```python
from build123d import *

# Parameters (mm, degrees)
F0_W     = 125
F0_H     = 75
F1_DEPTH = 2
F2_W     = 125
F2_H     = 2
F3_DEPTH = 40
F4_R     = 5
F5_R     = 5.08
F6_DEPTH = 100


with BuildPart() as f1:
    # F0 (on Front) → F1 (new body)
    with BuildSketch(Plane.XZ):
        Rectangle(F0_W, F0_H)
    extrude(amount=F1_DEPTH)

    # F2 (on face) → F3 (join)
    with BuildSketch(Plane.XZ.offset(2)):
        with Locations((0, -36.5)):
            Rectangle(F2_W, F2_H)
        with Locations((0, 36.5)):
            Rectangle(F2_W, F2_H)
    extrude(amount=F3_DEPTH)

    # F4
    f4_edges = [f1.edges().sort_by_distance(p)[0] for p in [
        (0, 0, 37.5),
        (0, 0, -37.5),
    ]]
    fillet(f4_edges, radius=F4_R)

    # F5 (on face) → F6 (cut)
    with BuildSketch(Plane.XY.offset(37.5)):
        with Locations((37.42, -25.08)):
            Circle(F5_R)
        with Locations((-37.42, -25.08)):
            Circle(F5_R)
    extrude(amount=-F6_DEPTH, mode=Mode.SUBTRACT)


solid = f1.part
```
Design review of the part built by this model. Coordinates are the model's own, in mm. A direction names the side the tool comes from. Give positions to 0.01 mm unless a question says otherwise; leave off trailing zeros. Write each loop counter-clockwise with the first axis right and the second up, starting at its lowest first coordinate (ties: lowest second). Pieces come first, ordered by that corner, then holes.
(1) Add section D-D (x = -2.5). Give the boundary of the cut face in (y, z), and give its area (3 significant figures).
Checked values:
outline: (-42, -37.5) - (-5, -37.5) arc R5 ccw to (0, -32.5) - (0, 32.5) arc R5 ccw to (-5, 37.5) - (-42, 37.5) - (-42, 35.5) - (-2, 35.5) - (-2, -35.5) - (-42, -35.5) - close
area: 299 mm2
(2) Tool access review of faces 4 (the face through (-1, -22, -35.5)), 5 (the face through (40.151, -20.797, -36.486)): name each direction out of +Z, -Z, +X, -X, +Y, -Y from which nothing blocks a thin tool from reaching the whole face with its end or side.
Checked values:
face 4: +X, -X, -Y
face 5: +Z, -Z
(3) Clearance check with flat-ended pins moving along their axes: pin 1 Ø13 at (x, y) = (-37.42, -25.08) entering from -Z; pin 2 Ø21.5 at (x, z) = (-22.5, -17) entering from -Y; pin 3 Ø8 at (x, y) = (-37.42, -25.08) entering from -Z. State where each tip first meets the part, or that it passes through.
Checked values:
pin 1: stops at z = -37.5
pin 2: stops at y = -2
pin 3: passes through
(4) Add section C-C (y = -32). Give the boundary of the cut face in (x, z), and give its area (3 significant figures).
Checked values:
outline: (-62.5, -37.5) - (62.5, -37.5) - (62.5, -35.5) - (-62.5, -35.5) - close; (-62.5, 35.5) - (62.5, 35.5) - (62.5, 37.5) - (-62.5, 37.5) - close
area: 500 mm2
(5) Mouldability with a two-part tool opening along X and no side actions: class faces 1 (the face through (-62.5, -1, 0)), 2 (the face through (-1, -2, 0)), 3 (the face through (-34.689, -20.797, -36.486)) as +X half, -X half, draft (parallel to the pull), parting line (faces both ways), or undercut.
Checked values:
face 1: -X half
face 2: draft
face 3: undercut
(6) Add section B-B (x = -37.42). Give the boundary of the cut face in (y, z).
Checked values:
outline: (-42, -37.5) - (-30.16, -37.5) - (-30.16, -35.5) - (-42, -35.5) - close; (-42, 35.5) - (-30.16, 35.5) - (-30.16, 37.5) - (-42, 37.5) - close; (-20, -37.5) - (-5, -37.5) arc R5 ccw to (0, -32.5) - (0, 32.5) arc R5 ccw to (-5, 37.5) - (-20, 37.5) - (-20, 35.5) - (-2, 35.5) - (-2, -35.5) - (-20, -35.5) - close
(7) Wall thickness on line 1 along Z through (x, y) = (-53.5, -22); line 2 along Y through (x, z) = (-32, -20); line 3 along Z through (x, y) = (-14.5, -4): over which ranges is each line inside the solid? List them lowest first.
Checked values:
line 1: z = -37.5 to -35.5, 35.5 to 37.5
line 2: y = -2 to 0
line 3: z = -37.4 to -35.5, 35.5 to 37.4
(8) Add section A-A (y = -25.08). Give the boundary of the cut face in (x, z).
Checked values:
outline: (-62.5, -37.5) - (-42.5, -37.5) - (-42.5, -35.5) - (-62.5, -35.5) - close; (-62.5, 35.5) - (-42.5, 35.5) - (-42.5, 37.5) - (-62.5, 37.5) - close; (-32.34, -37.5) - (32.34, -37.5) - (32.34, -35.5) - (-32.34, -35.5) - close; (-32.34, 35.5) - (32.34, 35.5) - (32.34, 37.5) - (-32.34, 37.5) - close; (42.5, -37.5) - (62.5, -37.5) - (62.5, -35.5) - (42.5, -35.5) - close; (42.5, 35.5) - (62.5, 35.5) - (62.5, 37.5) - (42.5, 37.5) - close
